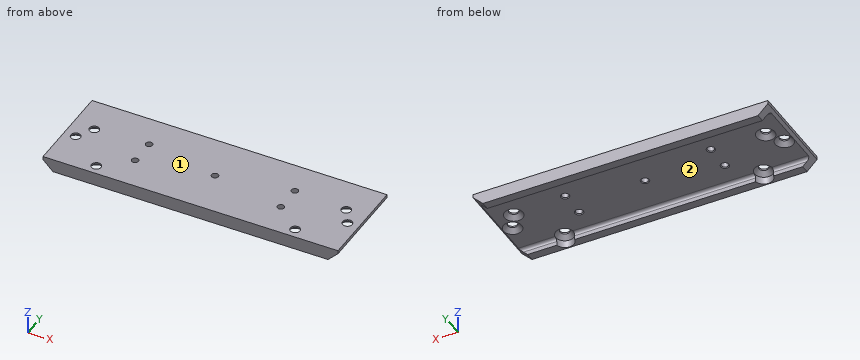
from build123d import *

# Parameters (mm, degrees)
SKETCH1_W                                      = 94
SKETCH1_H                                      = 28
BOSS_EXTRUDE1_DEPTH                            = 4
CHAMFER1_SIZE                                  = 5.5
CUT_EXTRUDE2_DEPTH                             = 48.772900268
CUT_EXTRUDE2_DEPTH_BACK                        = 48.772900268
SKETCH9_W                                      = 30.391833943
SKETCH9_H                                      = 28
SHELL1_START                                   = -11.5
SHELL1_DEPTH                                   = 23
FILLET1_R                                      = 1
CSK_FOR_M2_5_FLAT_HEAD_MACHINE_SCREW1_AT_COUNT = 2
CSK_FOR_M2_5_FLAT_HEAD_MACHINE_SCREW1_AT_PITCH = 5.830951895
CSK_FOR_M2_5_FLAT_HEAD_MACHINE_SCREW_2_COUNT   = 2
CSK_FOR_M2_5_FLAT_HEAD_MACHINE_SCREW_2_PITCH   = 16.124515497
SKETCH8_R                                      = 2.75
CUT_EXTRUDE1_DEPTH                             = 47.704523336
M2_5X0_45_TAPPED_HOLE1_D                       = 2.05
M2_5X0_45_TAPPED_HOLE1_DEPTH                   = 6
M2_5X0_45_TAPPED_HOLE1_CSINK_D                 = 2.55
M2_5X0_45_TAPPED_HOLE1_CSINK_ANGLE             = 90
M2_5X0_45_TAPPED_HOLE1_TIP                     = 0.615882135


# Read off the part's stored shape, not the designer's step: Shell1
with BuildPart() as part:
    # Sketch1 → Boss-Extrude1 (new body)
    with BuildSketch(Plane.XY):
        Rectangle(SKETCH1_W, SKETCH1_H)
    extrude(amount=BOSS_EXTRUDE1_DEPTH)

    # Chamfer1
    # the kernel refuses this chamfer: 5.5 mm, written as the material it takes off along each edge
    with BuildSketch(Plane(origin=(47, 28.144256434, 0), x_dir=(0.027495876610585942, 0, 0.9996219169112968), z_dir=(0, -1, 0)), Plane(origin=(-47, -28.144256434, 0), x_dir=(-0.027495876610585942, 0, 0.9996219169112968), z_dir=(0, 1, 0))) as chamfer1_piece_1:
        Polygon((CHAMFER1_SIZE * 0.999621916911, CHAMFER1_SIZE * 0.0274958766106), (-CHAMFER1_SIZE * 0.0274958766106, CHAMFER1_SIZE * 0.999621916911), (0, 0), align=None)
    extrude(amount=56.288512868, mode=Mode.SUBTRACT)

    # Sketch9 → Cut-Extrude2 (cut, two sides: drawn at the far end of the back side and taken through both)
    with BuildSketch(Plane(origin=(0, 0, 0), x_dir=(-1, 0, 0), z_dir=(0, 0, -1)).offset(-CUT_EXTRUDE2_DEPTH_BACK)):
        with Locations((-59.695916972, 0)):
            Rectangle(SKETCH9_W, SKETCH9_H)
        with Locations((59.695916972, 0)):
            Rectangle(SKETCH9_W, SKETCH9_H)
    extrude(amount=CUT_EXTRUDE2_DEPTH + CUT_EXTRUDE2_DEPTH_BACK, mode=Mode.SUBTRACT)

    # Shell1 outline → Shell1 (cut)
    with BuildSketch(Plane(origin=(0, 0, 0), x_dir=(1, 0, 0), z_dir=(0, 1, 0)).offset(SHELL1_START)):
        Polygon((-41.5, 0), (-43.75, -2.25), (43.75, -2.25), (41.5, 0), align=None)
    extrude(amount=SHELL1_DEPTH, mode=Mode.SUBTRACT)

    # Fillet1
    fillet1_edges = [part.edges().sort_by_distance(p)[0] for p in [
        (0, 11.5, 2.25),
        (0, -11.5, 2.25),
    ]]
    fillet(fillet1_edges, radius=FILLET1_R)

    # Sketch5 → CSK for M2.5 Flat Head Machine Screw1 (revolve, cut)
    with BuildSketch(Plane(origin=(38, 3, 2.25), x_dir=(0, 1, 0), z_dir=(1, 0, 0))):
        Polygon((0, 0), (0, 7.321247898), (1.45, 6.45), (1.45, 1.3), (2.75, 0), align=None)
    csk_for_m2_5_flat_head_machine_screw1 = revolve(axis=Axis((38, 3, -4.1), (0, 0, 1)), mode=Mode.SUBTRACT)

    # CSK for M2.5 Flat Head Machine Screw1 at: CSK for M2.5 Flat Head Machine Screw1 ×2
    with Locations(*[Vector(0.5144957554275275, -0.8574929257125438, 0) * (i * CSK_FOR_M2_5_FLAT_HEAD_MACHINE_SCREW1_AT_PITCH) for i in range(1, CSK_FOR_M2_5_FLAT_HEAD_MACHINE_SCREW1_AT_COUNT)]):
        add(csk_for_m2_5_flat_head_machine_screw1, mode=Mode.SUBTRACT)

    # CSK for M2.5 Flat Head Machine Screw 2: CSK for M2.5 Flat Head Machine Screw1 ×2
    with Locations(*[Vector(-0.4961389383568334, -0.8682431421244594, 0) * (i * CSK_FOR_M2_5_FLAT_HEAD_MACHINE_SCREW_2_PITCH) for i in range(1, CSK_FOR_M2_5_FLAT_HEAD_MACHINE_SCREW_2_COUNT)]):
        add(csk_for_m2_5_flat_head_machine_screw1, mode=Mode.SUBTRACT)

    # Sketch8 → Cut-Extrude1 (cut, through all)
    with BuildSketch(Plane(origin=(0, 0, 2.25), x_dir=(-1, 0, 0), z_dir=(0, 0, -1))):
        with Locations((-30, -11)):
            Circle(SKETCH8_R)
    cut_extrude1 = extrude(amount=CUT_EXTRUDE1_DEPTH, mode=Mode.SUBTRACT)

    # Mirror1: CSK for M2.5 Flat Head Machine Screw1, Cut-Extrude1 across plane
    add(csk_for_m2_5_flat_head_machine_screw1.mirror(Plane(origin=(0, 0, 0), x_dir=(0, 0, 1), z_dir=(1, 0, 0))), mode=Mode.SUBTRACT)
    add(cut_extrude1.mirror(Plane(origin=(0, 0, 0), x_dir=(0, 0, 1), z_dir=(1, 0, 0))), mode=Mode.SUBTRACT)

    # Mirror1 copy 1 sketch → Mirror1 copy 1 (revolve, cut)
    with BuildSketch(Plane(origin=(-41, -2, 2.25), x_dir=(0, 1, 0), z_dir=(-1, 0, 0))):
        Polygon((0, 0), (0, -7.321247898), (1.45, -6.45), (1.45, -1.3), (2.75, 0), align=None)
    revolve(axis=Axis((-41, -2, -4.1), (0, 0, -1)), mode=Mode.SUBTRACT)

    # Mirror1 copy 2 sketch → Mirror1 copy 2 (revolve, cut)
    with BuildSketch(Plane(origin=(-30, -11, 2.25), x_dir=(0, 1, 0), z_dir=(-1, 0, 0))):
        Polygon((0, 0), (0, -7.321247898), (1.45, -6.45), (1.45, -1.3), (2.75, 0), align=None)
    revolve(axis=Axis((-30, -11, -4.1), (0, 0, -1)), mode=Mode.SUBTRACT)

    # M2.5x0.45 Tapped Hole1
    with Locations(Plane(origin=(0, 0, 2.25), x_dir=(-1, 0, 0), z_dir=(0, 0, -1))):
        with Locations((0, 0), (-22, 4), (-22, -4), (22, -4), (22, 4)):
            CounterSinkHole(M2_5X0_45_TAPPED_HOLE1_D / 2, M2_5X0_45_TAPPED_HOLE1_CSINK_D / 2, depth=M2_5X0_45_TAPPED_HOLE1_DEPTH, counter_sink_angle=M2_5X0_45_TAPPED_HOLE1_CSINK_ANGLE)
            with Locations((0, 0, -(M2_5X0_45_TAPPED_HOLE1_DEPTH + M2_5X0_45_TAPPED_HOLE1_TIP / 2))):  # 118° drill point
                Cone(0, M2_5X0_45_TAPPED_HOLE1_D / 2, M2_5X0_45_TAPPED_HOLE1_TIP, mode=Mode.SUBTRACT)


solid = part.part
Could you check a few things on this model? Use its own coordinates, in mm. Face numbers are marked on the shaded views. Coordinates: 2 decimals unless noted, no trailing zeros. Loops run counter-clockwise (first coordinate to the right, second up) from the corner with the lowest first, then second, coordinate; pieces in that order, holes last.
1. Imagine slicing it at A-A (x = -30). Please give me the cut outline in (y, z), and give its area (3 significant figures).
2. I need wall thicknesses on L1, parallel to X at y = 4, z = 3.25 (3 decimals); L2, parallel to Y at x = -22, z = 3.1 (3 decimals); L3, parallel to X at y = -4, z = 3.3 (3 decimals). Which ranges of each line are inside material? Lowest first, please.
3. Imagine slicing it at B-B (x = 22). Please give me the cut outline in (y, z) (3 decimals), and give its area (3 significant figures).
4. For P1, Ø2.5, axis at x = 38, y = 3, coming from the +Z side; P2, Ø3.5, axis at x = 22, y = -4, coming from the -Z side; P3, Ø5, axis at x = -30, y = -11, coming from the +Z side; P4, Ø4, axis at x = 30, y = -11, coming from the -Z side, each with a flat end and sliding along its axis, tell me the tip position at first contact or that it passes through.
5. We'd pull the mould along Y, two halves only. Please class the marked faces 1 and 2: released by +Y, released by -Y, zero draft, split by the parting line, or undercut.
6. Imagine slicing it at C-C (x = -4.5). Please give me the cut outline in (y, z).
Computed values:
1. outline: (-14, 0) - (-13.75, 0) - (-13.75, 2.25) - (-12.45, 3.55) - (-12.45, 4) - (-14, 4) - close; (-9.55, 3.55) - (-8.25, 2.25) - (10.5, 2.25) arc R1 cw to (11.5, 1.25) - (11.5, 0) - (14, 0) - (14, 4) - (-9.55, 4) - close
1. area: 48.6 mm2
2. L1: x = -44.5 to -39.436, -36.564 to -23.025, -20.975 to 20.975, 23.025 to 36.564, 39.436 to 44.5
2. L2: y = -14 to -5.025, -2.975 to 2.975, 5.025 to 14
2. L3: x = -44.5 to -23.025, -20.975 to 20.975, 23.025 to 44.5
3. outline: (-14, 0) - (-11.5, 0) - (-11.5, 1.25) arc R1 cw to (-10.5, 2.25) - (-5.275, 2.25) - (-5.025, 2.5) - (-5.025, 4) - (-14, 4) - close; (-2.975, 2.5) - (-2.725, 2.25) - (2.725, 2.25) - (2.975, 2.5) - (2.975, 4) - (-2.975, 4) - close; (5.025, 2.5) - (5.275, 2.25) - (10.5, 2.25) arc R1 cw to (11.5, 1.25) - (11.5, 0) - (14, 0) - (14, 4) - (5.025, 4) - close
3. area: 53.4 mm2
4. P1: passes through
4. P2: stops at z = 2.25
4. P3: stops at z = 4
4. P4: stops at z = 3
5. face 1: zero draft
5. face 2: undercut
6. outline: (-14, 0) - (-11.5, 0) - (-11.5, 1.25) arc R1 cw to (-10.5, 2.25) - (10.5, 2.25) arc R1 cw to (11.5, 1.25) - (11.5, 0) - (14, 0) - (14, 4) - (-14, 4) - close
